```python
from build123d import *

# Parameters (mm, degrees)
SKETCH1_W           = 99.35
SKETCH1_H           = 37
BOSS_EXTRUDE1_DEPTH = 3.175
SKETCH2_W           = 2.8
SKETCH2_H           = 6
SKETCH2_H_2         = 8
CUT_EXTRUDE1_DEPTH  = 54.103071945
SKETCH3_W           = 79.35
SKETCH3_H           = 4
CUT_EXTRUDE2_DEPTH  = 54.103071945
FILLET1_R           = 3
FILLET2_R           = 0.5
SKETCH4_W           = 9.65
SKETCH4_H           = 3
CUT_EXTRUDE3_DEPTH  = 54.103071945
SKETCH5_W           = 12
SKETCH5_H           = 9
CUT_EXTRUDE4_DEPTH  = 54.103071945
FILLET3_R           = 0.5
FILLET4_R           = 0.5


with BuildPart() as part:
    # Sketch1 → Boss-Extrude1 (new body)
    with BuildSketch(Plane(origin=(0, 0, 0), x_dir=(0, 0, -1), z_dir=(1, 0, 0))):
        Rectangle(SKETCH1_W, SKETCH1_H)
    extrude(amount=BOSS_EXTRUDE1_DEPTH)

    # Sketch2 → Cut-Extrude1 (cut, through all)
    with BuildSketch(Plane(origin=(3.175, 0, 0), x_dir=(0, 0, -1), z_dir=(1, 0, 0))):
        with Locations((-46.275, 12.5)):
            Rectangle(SKETCH2_W, SKETCH2_H)
        with Locations((46.275, 12.5)):
            Rectangle(SKETCH2_W, SKETCH2_H)
        with Locations((-46.275, -7.325)):
            Rectangle(SKETCH2_W, SKETCH2_H_2)
        with Locations((46.275, -7.325)):
            Rectangle(SKETCH2_W, SKETCH2_H_2)
    extrude(amount=-CUT_EXTRUDE1_DEPTH, mode=Mode.SUBTRACT)

    # Sketch3 → Cut-Extrude2 (cut, through all)
    with BuildSketch(Plane(origin=(3.175, 0, 0), x_dir=(0, 0, -1), z_dir=(1, 0, 0))):
        with Locations((0, -16.5)):
            Rectangle(SKETCH3_W, SKETCH3_H)
    extrude(amount=-CUT_EXTRUDE2_DEPTH, mode=Mode.SUBTRACT)

    # Fillet1
    fillet1_edges = [part.edges().sort_by_distance(p)[0] for p in [
        (1.5875, -18.5, -49.675),
        (1.5875, -18.5, 49.675),
        (1.5875, -18.5, 39.675),
        (1.5875, -18.5, -39.675),
    ]]
    fillet(fillet1_edges, radius=FILLET1_R)

    # Fillet2
    fillet2_edges = [part.edges().sort_by_distance(p)[0] for p in [
        (1.5875, 18.5, 49.675),
        (1.5875, 18.5, -49.675),
        (1.5875, -14.5, 39.675),
        (1.5875, -14.5, -39.675),
    ]]
    fillet(fillet2_edges, radius=FILLET2_R)

    # Sketch4 → Cut-Extrude3 (cut, through all)
    with BuildSketch(Plane(origin=(3.175, 0, 0), x_dir=(0, 0, -1), z_dir=(1, 0, 0))):
        with Locations((0, 17)):
            Rectangle(SKETCH4_W, SKETCH4_H)
    extrude(amount=-CUT_EXTRUDE3_DEPTH, mode=Mode.SUBTRACT)

    # Sketch5 → Cut-Extrude4 (cut, through all)
    with BuildSketch(Plane(origin=(3.175, 0, 0), x_dir=(0, 0, -1), z_dir=(1, 0, 0))):
        with Locations((29.875, 1.775)):
            Rectangle(SKETCH5_W, SKETCH5_H)
    extrude(amount=-CUT_EXTRUDE4_DEPTH, mode=Mode.SUBTRACT)

    # Fillet3
    fillet3_edges = [part.edges().sort_by_distance(p)[0] for p in [
        (1.5875, -2.725, -23.875),
        (1.5875, 6.275, -23.875),
        (1.5875, 6.275, -35.875),
        (1.5875, -2.725, -35.875),
    ]]
    fillet(fillet3_edges, radius=FILLET3_R)

    # Fillet4
    fillet4_edges = [part.edges().sort_by_distance(p)[0] for p in [
        (1.5875, 18.5, 4.825),
        (1.5875, 18.5, -4.825),
    ]]
    fillet(fillet4_edges, radius=FILLET4_R)


solid = part.part
```
The model under review builds one solid part; all positions refer to its coordinate system, in mm. A direction names the side the tool comes from. Coordinates: 2 decimals unless noted, no trailing zeros. Write each loop counter-clockwise with the first axis right and the second up, starting at its lowest first coordinate (ties: lowest second). Pieces come first, ordered by that corner, then holes. Notation, with made-up numbers: (22, 3.5) - (78, 3.5) arc R20 cw to (78, 15.5) - close; hole circle Ø3 at (1.25, 54). An arc over 180 degrees is marked (long way). Answer in a Markdown table with one row per item. Add a question column.
Q1. Consider section D-D on x = 1. Give the number of separate pieces and of enclosed holes in the cut face, then the cut area to 3 significant figures.
Q2. Consider section C-C on z = -30.5. Give the boundary of the cut face in (x, y) (3 decimals), then the cut area to 3 significant figures.
Q3. Draft analysis for pull direction Z (two halves, no side actions). For faces 6 (the face through (1.61, -17.6, 48.82)), 7 (the face through (2, 18.5, 28)), 8 (the face through (2, 2, -23.875)), 9 (the face through (2, -14.5, 1)), state which applies: +Z half, -Z half, draft (parallel to the pull), parting line (faces both ways), or undercut.
Q4. Consider section A-A on y = 0. Give the boundary of the cut face in (x, z) (3 decimals).
Q5. Consider section B-B on y = -8. Give the boundary of the cut face in (x, z) (3 decimals).
Q6. Clearance check with a flat-ended pin moving along its axis: pin 1 (1.5 mm diameter, centred on x = 2, z = -34.5, fed in from -Y). State where the tip first meets the part, or that it passes through.
Q7. To check wall thickness, follow line 1 along Z through (x, y) = (2.45, -10) (3 decimals); line 2 along Y through (x, z) = (2.4, -25) (3 decimals); line 3 along Z through (x, y) = (1.75, -15) (3 decimals). State the ranges of each line that lie inside material, in increasing order. Write a range as from..to.
Q8. For faces 1 (the face through (3.175, 0, 1)), 2 (the face through (2, -18.5, -45)), 3 (the face through (1.565, -17.645, 40.577)), 4 (the face through (2, 2, -35.875)), 5 (the face through (2, 15.5, 0)), list the 3-axis set-ups (+Z, -Z, +X, -X, +Y, -Y) from which the entire face can be reached by the end or side of a thin tool; tool diameter is ignored.
Answers below:
| question | item | result |
|---|---|---|
| 1 | separate pieces | 1 |
| 1 | enclosed holes | 5 |
| 1 | area | 3,140 mm² |
| 2 | outline | (0, -14.5) - (3.175, -14.5) - (3.175, -2.725) - (0, -2.725) - close; (0, 6.275) - (3.175, 6.275) - (3.175, 18.5) - (0, 18.5) - close |
| 2 | area | 76.2 mm² |
| 3 | face 6 | +Z half |
| 3 | face 7 | draft |
| 3 | face 8 | undercut |
| 3 | face 9 | undercut |
| 4 | outline | (0, -49.675) - (3.175, -49.675) - (3.175, -35.875) - (0, -35.875) - close; (0, -23.875) - (3.175, -23.875) - (3.175, 49.675) - (0, 49.675) - close |
| 5 | outline | (0, -49.675) - (3.175, -49.675) - (3.175, -47.675) - (0, -47.675) - close; (0, -44.875) - (3.175, -44.875) - (3.175, 44.875) - (0, 44.875) - close; (0, 47.675) - (3.175, 47.675) - (3.175, 49.675) - (0, 49.675) - close |
| 6 | pin 1 | y = -14.5 |
| 7 | line 1 | -49.675..-47.675, -44.875..44.875, 47.675..49.675 |
| 7 | line 2 | -14.5..-2.725, 6.275..18.5 |
| 7 | line 3 | -49.675..-39.675, 39.675..49.675 |
| 8 | face 1 | +Z, -Z, +X, +Y, -Y |
| 8 | face 2 | +Z, -Z, +X, -X, -Y |
| 8 | face 3 | +X, -X, -Y |
| 8 | face 4 | +X, -X |
| 8 | face 5 | +X, -X, +Y |
